Can you work these out from the model? Positions are in its coordinate system, mm. A direction names the side the tool comes from. Give positions to 0.01 mm unless a question says otherwise; leave off trailing zeros. Order: outer loops, then holes, each group sorted by start corner. A loop starts at its lowest first (then second) coordinate and runs counter-clockwise, first axis right, second up. Notation, with made-up numbers: (-25, 57.25) -> (-4, 57.25) arc R13 ccw to (-4, 73.25) -> close; hole circle Ø9 at (-19, 75.25). An arc over 180 degrees is marked (long way). Answer as a JSON object with one key per item and string values.
Autodesk Inventor part; units mm, degrees
ref_plane "YZ Plane" through (0, 0, 0) normal (1, 0, 0) x (0, 1, 0)
ref_plane "XZ Plane" through (0, 0, 0) normal (0, 1, 0) x (-1, 0, 0)
ref_plane "XY Plane" through (0, 0, 0) normal (0, 0, 1) x (1, 0, 0)
sketch "Náčrt1" plane through (0, 0, 0) normal (0, 1, 0) x (-1, 0, 0)
  line L0 (7.7382, 6.9283) -> (7.7382, -42.0717)
  line L1 (7.7382, -42.0717) -> (-31.2618, -42.0717)
  line L2 (-31.2618, -42.0717) -> (-31.2618, 6.9283)
  line L3 (-31.2618, 6.9283) -> (7.7382, 6.9283)
  line L4 (6.7382, -41.0717) -> (6.7382, 5.9283)
  line L5 (6.7382, 5.9283) -> (-30.2618, 5.9283)
  line L6 (-30.2618, 5.9283) -> (-30.2618, -41.0717)
  line L7 (-30.2618, -41.0717) -> (6.7382, -41.0717)
  point P0 (0, 0)
  dimension "d0" = 49
  dimension "d1" = 39
  dimension "d2" = 1
extrude "Vysunutí1" add sketch "Náčrt1" along normal blind 15
sketch "Náčrt2" plane through (0, 15, 0) normal (0, 1, 0) x (1, 0, 0)
  line L0 (31.2618, -6.9283) -> (31.2618, 42.0717)
  line L1 (31.2618, 42.0717) -> (-7.7382, 42.0717)
  line L2 (-7.7382, 42.0717) -> (-7.7382, -6.9283)
  line L3 (-7.7382, -6.9283) -> (31.2618, -6.9283)
  line L4 (-6.7382, 41.0717) -> (30.2618, 41.0717)
  line L5 (30.2618, 41.0717) -> (30.2618, -5.9283)
  line L6 (30.2618, -5.9283) -> (-6.7382, -5.9283)
  line L7 (-6.7382, -5.9283) -> (-6.7382, 41.0717)
  line L8 (-7.7382, -6.9283) -> (31.2618, -6.9283)
  line L9 (31.2618, -6.9283) -> (31.2618, 42.0717)
  line L10 (31.2618, 42.0717) -> (-7.7382, 42.0717)
  line L11 (-7.7382, 42.0717) -> (-7.7382, -6.9283)
  point P0 (0, 0)
extrude "Vysunutí2" add sketch "Náčrt2" along normal blind 1 contours L3 L2 L1 L0 | L4 L5 L6 L7
sketch "Náčrt3" plane through (31.2618, 0, 6.9283) normal (1, 0, 0) x (0, 0, -1)
  line L0 (0, 0) -> (49, 0)
  line L1 (49, 0) -> (49, 16)
  line L2 (0, 16) -> (49, 16)
  line L3 (0, 0) -> (0, 16)
  line L4 (0, 0) -> (49, 0)
  line L5 (49, 0) -> (49, 6)
  line L6 (49, 6) -> (0, 6)
  line L7 (0, 6) -> (0, 0)
  point P0 (6.9283, 0)
  point P1 (0, 6)
  dimension "d7" = 6
extrude "Vysunutí3" cut sketch "Náčrt3" against normal blind 1 contours L3 L6 L1 L0
sketch "Náčrt4" plane through (31.2618, 16, 6.9283) normal (1, 0, 0) x (0, 0, -1)
  line L0 (0, -10) -> (49, -10)
  line L1 (49, -10) -> (49, 0)
  line L2 (0, 0) -> (49, 0)
  line L3 (0, -10) -> (0, 0)
  line L4 (20, -10) -> (29, -10)
  line L5 (29, -10) -> (29, -9)
  line L6 (29, -9) -> (20, -9)
  line L7 (20, -9) -> (20, -10)
  point P0 (6.9283, -16)
  dimension "d10" = 20
  dimension "d11" = 1
  dimension "d12" = 20
extrude "Vysunutí4" add sketch "Náčrt4" along normal blind 15 contours L7 L6 L5 L0
properties part number "Víko senzor"
1. Please list where these lines run through material, in increasing order: L1, parallel to Z at x = 0.5, y = 7.5; L2, parallel to X at y = 12.25, z = -6; L3, parallel to Y at x = 11, z = -7.
Worked answers:
{"L1": "-42.07 to -41.07, 5.93 to 6.93", "L2": "-7.74 to -6.74, 30.26 to 31.26", "L3": "15 to 16"}
2. Will these pins go through, and if not, where does the flat tip stop? pin 1 Ø18.5 at (x, z) = (6, -13.5) entering from -Y; pin 2 Ø2.5 at (x, z) = (40.5, -17) entering from +Y; pin 3 Ø17.5 at (x, z) = (40.5, -6) entering from -Y.
Worked answers:
{"pin 1": "y = 15", "pin 2": "y = 7", "pin 3": "y = 6"}
3. If we section it at D-D on y = 4: Please give me the cut outline in (x, z), then the cut area to 3 significant figures.
Worked answers:
{"outline": "(-7.74, -42.07) -> (30.26, -42.07) -> (30.26, -41.07) -> (-6.74, -41.07) -> (-6.74, 5.93) -> (30.26, 5.93) -> (30.26, 6.93) -> (-7.74, 6.93) -> close", "area": "123 mm²"}
4. If we section it at A-A on y = 14: Please give me the cut outline in (x, z).
Worked answers:
{"outline": "(-7.74, -42.07) -> (31.26, -42.07) -> (31.26, 6.93) -> (-7.74, 6.93) -> close; hole (-6.74, -41.07) -> (30.26, -41.07) -> (30.26, 5.93) -> (-6.74, 5.93) -> close"}
5. For faces 1 (the face through (30.262, 10, -17)), 2 (the face through (39, 7, -18)), 3 (the face through (37, 6, -18)), 4 (the face through (-7, 0, -7)), 5 (the face through (11, 8, -42.072)), which set-ups out of +Z, -Z, +X, -X, +Y, -Y let a thin tool reach every point of the face, with its end or its side?
Worked answers:
{"face 1": "-Y", "face 2": "+Z, -Z, +X, +Y", "face 3": "+Z, -Z, +X, -Y", "face 4": "+Z, -Z, +X, -X, -Y", "face 5": "-Z, +X, -X, +Y, -Y"}
6. If we section it at C-C on x = 8: Please give me the cut outline in (y, z), then the cut area to 3 significant figures.
Worked answers:
{"outline": "(0, -42.07) -> (16, -42.07) -> (16, 6.93) -> (0, 6.93) -> (0, 5.93) -> (15, 5.93) -> (15, -41.07) -> (0, -41.07) -> close", "area": "79.0 mm²"}
7. If we section it at B-B on z = -20: Please give me the cut outline in (x, y).
Worked answers:
{"outline": "(-7.74, 0) -> (-6.74, 0) -> (-6.74, 15) -> (30.26, 15) -> (30.26, 6) -> (46.26, 6) -> (46.26, 7) -> (31.26, 7) -> (31.26, 16) -> (-7.74, 16) -> close"}
8. If we mould it in two halves opening along X, with no side actions, what happens to faces 6 (the face through (-6.738, 7, -18)), 7 (the face through (12, 7, -41.072)), 8 (the face through (-7.738, 8, -17)), 9 (the face through (12, 8, 6.928))? For each: +X half, -X half, draft (parallel to the pull), parting line (faces both ways), or undercut.
Worked answers:
{"face 6": "undercut", "face 7": "undercut", "face 8": "-X half", "face 9": "draft"}
